from build123d import *

# Parameters (mm, degrees)
SKETCH1_W           = 50.8
SKETCH1_H           = 50.8
BOSS_EXTRUDE1_DEPTH = 6.35
CUT_EXTRUDE1_DEPTH  = 6.35


with BuildPart() as part:
    # Sketch1 → Boss-Extrude1 (new body)
    with BuildSketch(Plane(origin=(0, 0, 0), x_dir=(1, 0, 0), z_dir=(0, 1, 0))):
        with Locations((25.4, 25.4)):
            Rectangle(SKETCH1_W, SKETCH1_H)
    extrude(amount=BOSS_EXTRUDE1_DEPTH)

    # Sketch2 → Cut-Extrude1 (cut)
    with BuildSketch(Plane(origin=(0, 6.35, 0), x_dir=(1, 0, 0), z_dir=(0, 1, 0))):
        Polygon((28.575, 28.575), (40.216666667, 28.575), (40.216666667, 22.225), (28.575, 22.225), (28.575, 10.583333333), (22.225, 10.583333333), (22.225, 22.225), (10.583333333, 22.225), (10.583333333, 28.575), (22.225, 28.575), (22.225, 40.216666667), (28.575, 40.216666667), align=None)
    extrude(amount=-CUT_EXTRUDE1_DEPTH, mode=Mode.SUBTRACT)


solid = part.part
Geometry: final body of the model. Coordinates: model frame, mm. A direction names the side the tool comes from. Coordinates: 2 decimals unless noted, no trailing zeros. Order: outer loops, then holes, each group sorted by start corner. A loop starts at its lowest first (then second) coordinate and runs counter-clockwise, first axis right, second up.
(1) Section query B-B (z = -39). Return the cut outline in (x, y) (3 decimals).
(2) Material intervals for probe 1 along Z at (x, y) = (34, 2) (3 decimals); probe 2 along X at (y, z) = (4.5, -14) (3 decimals); probe 3 along X at (y, z) = (2.25, -28), sorted ascending.
(3) Section query A-A (x = 24). Return the cut outline in (y, z), plus the area to 3 significant figures.
(4) Access query for faces 1 (the face through (22.225, 3, -34)), 2 (the face through (31, 6.35, -20)). Directions: +Z, -Z, +X, -X, +Y, -Y. A direction counts if a zero-diameter tool reaches every point of the face in a straight line with its end or side. Return the directions, or none.
(5) Section query C-C (y = 4). Return the cut outline in (x, z) (3 decimals), plus the area to 3 significant figures.
(6) Draft query along Z for faces 3 (the face through (16, 3, -22.225)), 4 (the face through (0, 3, -25)), 5 (the face through (25, 3, 0)). Return one class per face: pulls with the +Z half, pulls with the -Z half, needs draft (parallel to the pull), parting line crosses it, or undercut.
Solution:
1. outline: (0, 0) - (22.225, 0) - (22.225, 6.35) - (0, 6.35) - close; (28.575, 0) - (50.8, 0) - (50.8, 6.35) - (28.575, 6.35) - close
2. probe 1: z = -50.8 to -28.575, -22.225 to 0
2. probe 2: x = 0 to 22.225, 28.575 to 50.8
2. probe 3: x = 0 to 10.58, 40.22 to 50.8
3. outline: (0, -50.8) - (6.35, -50.8) - (6.35, -40.22) - (0, -40.22) - close; (0, -10.58) - (6.35, -10.58) - (6.35, 0) - (0, 0) - close
3. area: 134 mm2
4. face 1: +Y, -Y
4. face 2: +Z, -Z, +X, -X, +Y
5. outline: (0, -50.8) - (50.8, -50.8) - (50.8, 0) - (0, 0) - close; hole (10.583, -28.575) - (22.225, -28.575) - (22.225, -40.217) - (28.575, -40.217) - (28.575, -28.575) - (40.217, -28.575) - (40.217, -22.225) - (28.575, -22.225) - (28.575, -10.583) - (22.225, -10.583) - (22.225, -22.225) - (10.583, -22.225) - close
5. area: 2,240 mm2
6. face 3: undercut
6. face 4: needs draft
6. face 5: pulls with the +Z half
